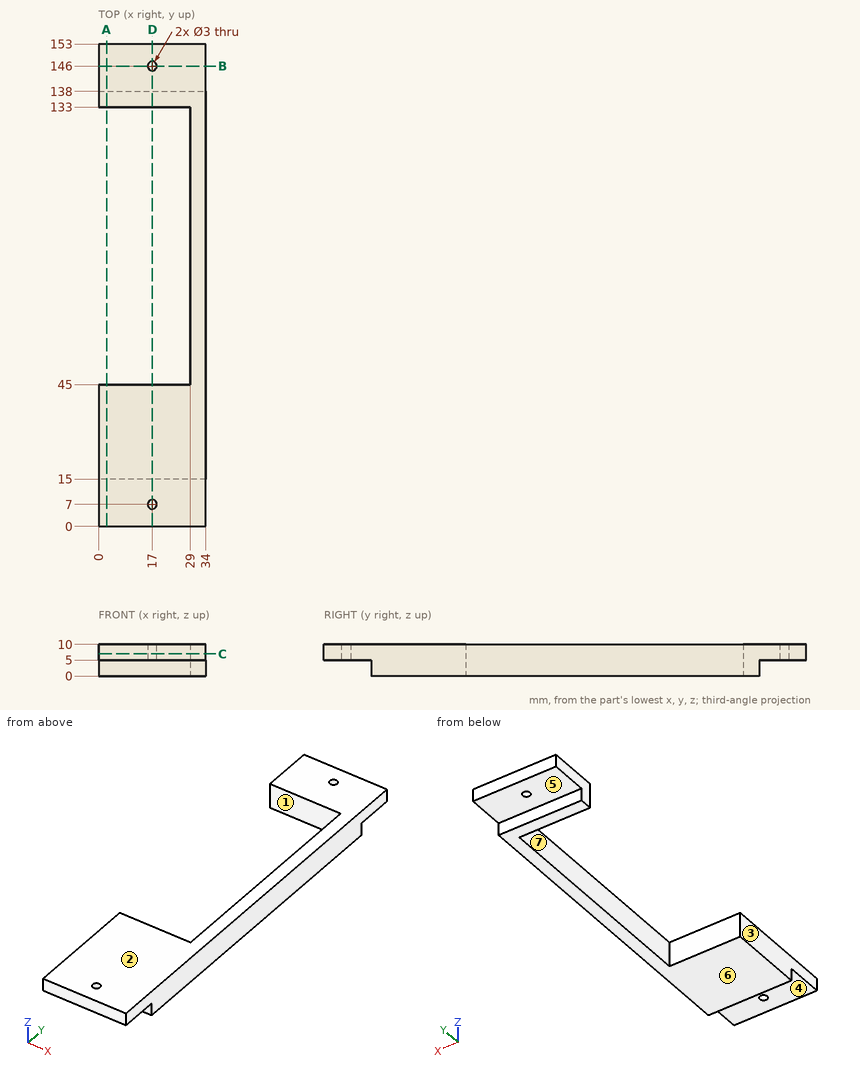
Verification items for this drawing (mm, ordinates from the low corner). A direction names the side the tool comes from. Round coordinates to 2 decimals unless told otherwise and drop trailing zeros. Order: outer loops, then holes, each group sorted by start corner. A loop starts at its lowest first (then second) coordinate and runs counter-clockwise, first axis right, second up. Notation, with made-up numbers: (74.25, 35.5) - (113.25, 35.5) arc R18 cw to (113.25, 59.5) - close; hole circle Ø10 at (-11, 57). An arc over 180 degrees is marked (long way). Answer as CSV lines item,"result". Start each with the question number.
1) Depth check by flat-ended pin: pin 1 (10 mm diameter, centred on x = 10.5, y = 132.5, fed in from +Z); pin 2 (4 mm diameter, centred on y = 48.5, z = 3.5, fed in from -X); pin 3 (1.5 mm diameter, centred on x = 15, z = 3, fed in from -Y); pin 4 (7.5 mm diameter, centred on x = 22, y = 5.5, fed in from -Z). Enter the tip coordinate at first touch or a pass-through.
2) Scan lines: probe 1 along Y at (x, z) = (17, 8); probe 2 along Y at (x, z) = (5, 6.5); probe 3 along Y at (x, z) = (7.5, 4). Record each from-to range of solid material in increasing order.
3) Tool access check on the marked faces 1, 2, 3, 4 and 5. Record the directions out of +Z, -Z, +X, -X, +Y, -Y that give a thin tool (end or side, any length) a straight path to the whole face; none if there is none.
4) Section check C-C (z = 7). Record the cut outline in (x, y).
5) Section check B-B (y = 146). Record the cut outline in (x, z).
6) Section check D-D (x = 17). Record the cut outline in (y, z), then the cut area to 3 significant figures.
7) Draft check along Y on the marked faces 6 and 7. Enter one of: +Y half, -Y half, draft (parallel to the pull), parting line (faces both ways), or undercut.
8) Section check A-A (x = 2.5). Record the cut outline in (y, z), then the cut area to 3 significant figures.
Determined:
1,pin 1,"z = 10"
1,pin 2,"x = 29"
1,pin 3,"y = 15"
1,pin 4,"z = 5"
2,probe 1,"0 to 5.5, 8.5 to 45, 133 to 144.5, 147.5 to 153"
2,probe 2,"0 to 45, 133 to 153"
2,probe 3,"15 to 45, 133 to 138"
3,face 1,"+Z, -Z, -X"
3,face 2,"+Z, +X, -X, +Y, -Y"
3,face 3,"+Z, -Z, -X, +Y, -Y"
3,face 4,"-Z, +X, -X, -Y"
3,face 5,"-Z, +X, -X, +Y"
4,outline,"(0, 0) - (34, 0) - (34, 153) - (0, 153) - (0, 133) - (29, 133) - (29, 45) - (0, 45) - close; hole circle Ø3 at (17, 7); hole circle Ø3 at (17, 146)"
5,outline,"(0, 5) - (15.5, 5) - (15.5, 10) - (0, 10) - close; (18.5, 5) - (34, 5) - (34, 10) - (18.5, 10) - close"
6,outline,"(0, 5) - (5.5, 5) - (5.5, 10) - (0, 10) - close; (8.5, 5) - (15, 5) - (15, 0) - (45, 0) - (45, 10) - (8.5, 10) - close; (133, 0) - (138, 0) - (138, 5) - (144.5, 5) - (144.5, 10) - (133, 10) - close; (147.5, 5) - (153, 5) - (153, 10) - (147.5, 10) - close"
6,area,"470 mm^2"
7,face 6,"draft"
7,face 7,"undercut"
8,outline,"(0, 5) - (15, 5) - (15, 0) - (45, 0) - (45, 10) - (0, 10) - close; (133, 0) - (138, 0) - (138, 5) - (153, 5) - (153, 10) - (133, 10) - close"
8,area,"500 mm^2"
